The listing builds one solid part. Answer for the finished solid, in the listing's coordinates (mm). Round coordinates to 2 decimals unless told otherwise and drop trailing zeros. Order: outer loops, then holes, each group sorted by start corner. A loop starts at its lowest first (then second) coordinate and runs counter-clockwise, first axis right, second up. Notation, with made-up numbers: (-15, 13) - (10, 13) arc R19 cw to (10, 29) - close; hole circle Ø7 at (-13.75, -26.5). An arc over 180 degrees is marked (long way). One line per item, written item: value. Start each with the question number.
1. Section D-D, the plane z = 7.5 is taken. Give the vertices of the cut face in (x, y) (3 decimals), then the cut area to 3 significant figures.
2. A straight line is drawn through the part: line 1 (Y direction, x = 28, z = 28) (3 decimals). Find the intervals that lie inside material, in ascending order.
3. For a pull along Y with two mould halves and no side action, classify faces 1 (the cylindrical face through (1.565, 17.503, 29.195)), 2 (the flat face through (20, 3.175, 19)), 3 (the flat face through (3.175, 21, 19)) as released by +Y, released by -Y, zero draft, split by the parting line, or undercut.
4. Section C-C, the plane x = 27.5 is taken. Give the vertices of the cut face in (y, z) (3 decimals), then the cut area to 3 significant figures.
5. Section A-A, the plane y = 18 is taken. Give the vertices of the cut face in (x, z) (3 decimals).
6. Flat-ended cylindrical pins translate along their axes: P1, Ø6, axis at x = 31, z = 22.5, coming from the +Y side (3 decimals); P2, Ø17.5, axis at y = 23, z = 27.5, coming from the +X side (3 decimals); P3, Ø1.5, axis at y = 21, z = 33, coming from the -X side; P4, Ø5.5, axis at y = 22.225, z = 28.575, coming from the -X side. Find the tip coordinate at first contact, or state that the pin passes through.
7. Section B-B, the plane z = 27 is taken. Give the vertices of the cut face in (x, y) (3 decimals).
Autodesk Inventor part; units mm, degrees
ref_plane "YZ Plane" through (0, 0, 0) normal (1, 0, 0) x (0, 1, 0)
ref_plane "XZ Plane" through (0, 0, 0) normal (0, 1, 0) x (-1, 0, 0)
ref_plane "XY Plane" through (0, 0, 0) normal (0, 0, 1) x (1, 0, 0)
sketch "Sketch1" plane through (0, 0, 0) normal (0, 0, 1) x (1, 0, 0)
  line L0 (0, 0) -> (0, 38.1)
  line L1 (0, 38.1) -> (3.175, 38.1)
  line L2 (3.175, 38.1) -> (3.175, 3.175)
  line L3 (3.175, 3.175) -> (38.1, 3.175)
  line L4 (38.1, 3.175) -> (38.1, 0)
  line L5 (38.1, 0) -> (0, 0)
  dimension "d0" = 38.1
  dimension "d1" = 3.175
extrude "Extrusion1" add sketch "Sketch1" along normal blind 38.1
sketch "Sketch2" plane through (3.175, 3.175, 0) normal (1, 0, 0) x (0, 0, -1)
  line L0 (0, 34.925) -> (-38.1, 34.925)
  line L1 (-38.1, 0) -> (-38.1, 34.925)
  line L2 (0, 0) -> (-38.1, 0)
  point P0 (0, -3.175)
  point P1 (-28.575, 19.05)
  dimension "d5" = 9.525
  dimension "d24" = 19.05
hole "Hole1" at (3.175, 22.225, 28.575) direction (-1, 0, 0) diameter 9.525 end through all
sketch "Sketch3" plane through (3.175, 3.175, 0) normal (0, 1, 0) x (1, 0, 0)
  line L0 (34.925, -38.1) -> (0, -38.1)
  line L1 (0, 0) -> (0, -38.1)
  line L2 (34.925, 0) -> (34.925, -38.1)
  point P0 (-3.175, 0)
  point P1 (8.9154, -28.1686)
  point P2 (23.3172, -12.8778)
  dimension "d13" = 9.9314
  dimension "d14" = 8.9154
  dimension "d15" = 25.2222
  dimension "d16" = 11.6078
hole "Hole2" at (12.0904, 3.175, 28.1686) at (26.4922, 3.175, 12.8778) direction (0, -1, 0) diameter 5.1054 end through all
properties part number "CLB_085_ClimberMountLBracket" material "Aluminum 6061"
Answer list:
1. outline: (0, 0) - (38.1, 0) - (38.1, 3.175) - (3.175, 3.175) - (3.175, 38.1) - (0, 38.1) - close
1. area: 232 mm²
2. line 1: y = 0 to 3.175
3. face 1: undercut
3. face 2: released by +Y
3. face 3: zero draft
4. outline: (0, 0) - (3.175, 0) - (3.175, 10.532) - (0, 10.532) - close; (0, 15.223) - (3.175, 15.223) - (3.175, 38.1) - (0, 38.1) - close
4. area: 106 mm²
5. outline: (0, 0) - (3.175, 0) - (3.175, 26.377) - (0, 26.377) - close; (0, 30.773) - (3.175, 30.773) - (3.175, 38.1) - (0, 38.1) - close
6. P1: stops at y = 3.175
6. P2: stops at x = 3.175
6. P3: stops at x = 0
6. P4: passes through
7. outline: (0, 0) - (9.821, 0) - (9.821, 3.175) - (3.175, 3.175) - (3.175, 17.73) - (0, 17.73) - close; (0, 26.72) - (3.175, 26.72) - (3.175, 38.1) - (0, 38.1) - close; (14.36, 0) - (38.1, 0) - (38.1, 3.175) - (14.36, 3.175) - close
